Build history of the part. All positions in model axes, mm. A direction names the side the tool comes from. Give positions to 0.01 mm unless a question says otherwise; leave off trailing zeros. Order: outer loops, then holes, each group sorted by start corner. A loop starts at its lowest first (then second) coordinate and runs counter-clockwise, first axis right, second up. Notation, with made-up numbers: M 52.25,-16 L 70.25,-16 A25 ccw 70.25,1 Z; hole C 62.25,85 d5. An arc over 180 degrees is marked long. One line per item, written item: value.
Autodesk Inventor part; units mm, degrees
ref_plane "YZ Plane" through (0, 0, 0) normal (1, 0, 0) x (0, 1, 0)
ref_plane "XZ Plane" through (0, 0, 0) normal (0, 1, 0) x (-1, 0, 0)
ref_plane "XY Plane" through (0, 0, 0) normal (0, 0, 1) x (1, 0, 0)
sketch "Náčrt1" plane through (0, 0, 0) normal (0, 0, 1) x (1, 0, 0)
  line L0 (-70, 0) -> (70, 0)
  line L1 (0, -49) -> (0, 49)
  line L2 (-50, 35) -> (50, 35)
  line L3 (50, 35) -> (50, -35)
  line L4 (50, -35) -> (-50, -35)
  line L5 (-50, -35) -> (-50, 35)
  point P0 (0, 0)
  point P1 (0, 35)
  point P2 (-50, 0)
  dimension "d0" = 70
  dimension "d1" = 100
extrude "Vysunutí1" add sketch "Náčrt1" along normal blind 10
fillet "Zaoblení1" radius 5 4 edges at (50, 35, 5) (50, -35, 5) (-50, -35, 5) (-50, 35, 5)
sketch "Náčrt2" plane through (0, 0, 10) normal (0, 0, 1) x (1, 0, 0)
  line L0 (-50, 30) -> (-50, -30)
  point P0 (0, 0)
  point P1 (-27.5, 17.5)
  point P2 (-27.5, -17.5)
  point P3 (-50, 0)
  dimension "d5" = 22.5
  dimension "d6" = 22.5
  dimension "d7" = 35
  dimension "d8" = 17.5
hole "Díra1" at (-27.5, 17.5, 10) at (-27.5, -17.5, 10) direction (0, 0, -1) diameter 9 end through all
sketch "Náčrt3" plane through (0, 0, 10) normal (0, 0, 1) x (1, 0, 0)
  line L0 (50, -30) -> (50, 30)
  line L1 (37.5, 22.5) -> (22.5, 22.5) construction
  line L2 (37.5, 26) -> (22.5, 26)
  line L3 (22.5, 19) -> (37.5, 19)
  arc A0 (37.5, 19) -> (37.5, 26) centre (37.5, 22.5) ccw
  arc A1 (22.5, 26) -> (22.5, 19) centre (22.5, 22.5) ccw
  line L4 (37.5, -22.5) -> (22.5, -22.5) construction
  line L5 (37.5, -19) -> (22.5, -19)
  line L6 (22.5, -26) -> (37.5, -26)
  arc A2 (37.5, -26) -> (37.5, -19) centre (37.5, -22.5) ccw
  arc A3 (22.5, -19) -> (22.5, -26) centre (22.5, -22.5) ccw
  point P0 (0, 0)
  point P1 (50, 0)
  point P2 (30, 22.5)
  point P3 (30, -22.5)
  dimension "d16" = 45
  dimension "d17" = 22.5
  dimension "d18" = 12.5
  dimension "d19" = 12.5
  dimension "d20" = 15
  dimension "d21" = 7
  dimension "d22" = 15
  dimension "d23" = 7
hole "Díra2" at (37.5, 22.5, 10) at (37.5, -22.5, 10) direction (0, 0, -1) diameter 3.4 end through all
extrude "Vysunutí2" cut sketch "Náčrt3" against normal blind 4
sketch "Náčrt4" plane through (0, 0, 10) normal (0, 0, 1) x (1, 0, 0)
  circle A0 centre (37.5, 22.5) radius 1.7
  arc A1 (22.5, 26) -> (22.5, 19) centre (22.5, 22.5) ccw
  line L0 (37.5, 22.5) -> (22.5, 22.5) construction
  line L1 (37.5, 20.8) -> (22.5, 20.8)
  line L2 (22.5, 24.2) -> (37.5, 24.2)
  arc A2 (37.5, 20.8) -> (37.5, 24.2) centre (37.5, 22.5) ccw
  arc A3 (22.5, 24.2) -> (22.5, 20.8) centre (22.5, 22.5) ccw
  circle A4 centre (37.5, -22.5) radius 1.7
  line L3 (37.5, -22.5) -> (22.5, -22.5) construction
  line L4 (37.5, -24.2) -> (22.5, -24.2)
  line L5 (22.5, -20.8) -> (37.5, -20.8)
  arc A5 (37.5, -24.2) -> (37.5, -20.8) centre (37.5, -22.5) ccw
  arc A6 (22.5, -20.8) -> (22.5, -24.2) centre (22.5, -22.5) ccw
  arc A7 (22.5, -19) -> (22.5, -26) centre (22.5, -22.5) ccw
  point P0 (0, 0)
  point P1 (30, 22.5)
  point P2 (30, -22.5)
extrude "Vysunutí3" cut sketch "Náčrt4" against normal through all
properties part number "drzal_kamery_real_sense"
1) Drill centre lines: probe 1 along Y at (x, z) = (30.5, 3.25); probe 2 along Y at (x, z) = (-27.5, 3.75); probe 3 along X at (y, z) = (-17.5, 2.5). Where is each one in solid material? Low to high. Write a range as from..to.
Check values:
probe 1: -35..-24.2, -20.8..20.8, 24.2..35
probe 2: -35..-22, -13..13, 22..35
probe 3: -50..-32, -23..50
2) Saw through at D-D, the plane y = -15. Write the cut outline in (x, z).
Check values:
outline: M -50,0 L -31.24,0 L -31.24,10 L -50,10 Z; M -23.76,0 L 50,0 L 50,10 L -23.76,10 Z
3) Saw through at B-B, the plane z = 7.5. Write the cut outline in (x, y).
Check values:
outline: M -50,-30 A5 ccw -45,-35 L 45,-35 A5 ccw 50,-30 L 50,30 A5 ccw 45,35 L -45,35 A5 ccw -50,30 Z; hole C -27.5,-17.5 d9; hole C -27.5,17.5 d9; hole M 22.5,-26 L 37.5,-26 A3.5 ccw 37.5,-19 L 22.5,-19 A3.5 ccw Z; hole M 22.5,19 L 37.5,19 A3.5 ccw 37.5,26 L 22.5,26 A3.5 ccw Z
4) Saw through at A-A, the plane y = 17.5. Write the cut outline in (x, z), then the cut area to 3 significant figures.
Check values:
outline: M -50,0 L -32,0 L -32,10 L -50,10 Z; M -23,0 L 50,0 L 50,10 L -23,10 Z
area: 910 mm^2
5) Tool access for faces 4 (the face through (41, 22.4, 8)), 5 (the face through (30, 24.2, 3)), 6 (the face through (-1, 0, 0)): list every direction of +Z, -Z, +X, -X, +Y, -Y with a clear straight run to the whole face (end or side of a thin tool).
Check values:
face 4: +Z
face 5: +Z, -Z
face 6: -Z, +X, -X, +Y, -Y
6) Pin check, flat tip, straight feed: pin 1 (3.5 mm diameter, centred on x = 32.5, y = 22.5, fed in from +Z). Stop position of the tip, or through.
Check values:
pin 1: z = 6
7) Saw through at C-C, the plane x = 28. Write the cut outline in (y, z).
Check values:
outline: M -35,0 L -24.2,0 L -24.2,6 L -26,6 L -26,10 L -35,10 Z; M -20.8,0 L 20.8,0 L 20.8,6 L 19,6 L 19,10 L -19,10 L -19,6 L -20.8,6 Z; M 24.2,0 L 35,0 L 35,10 L 26,10 L 26,6 L 24.2,6 Z
8) Mould opens along Y. For faces 1 (the face through (-1, 0, 10)), 2 (the face through (48, -34, 5)), 3 (the face through (19, 22.6, 8)) say: released by +Y, released by -Y, zero draft, split by the parting line, or undercut.
Check values:
face 1: zero draft
face 2: released by -Y
face 3: undercut
